```python
from build123d import *

# Parameters (mm, degrees)
F2_R     = 12.7
F3_DEPTH = 4.7625
F4_SIZE  = 1.27


with BuildPart() as f1:
    # F0 (on Front) → F1 (revolve)
    with BuildSketch(Plane.XZ):
        Polygon((-4.7625, 0), (0, 0), (0, 50.8), (-10.16, 50.8), (-10.16, 46.0375), (-4.7625, 46.0375), align=None)
    revolve(axis=Axis((0, 0, 25.4), (0, 0, -1)))

    # F2 (on face) → F3 (cut, through all)
    with BuildSketch(Plane.XY.offset(50.8)):
        Circle(F2_R)
        Polygon((-8.798818, 5.08), (0, 10.16), (8.798818, 5.08), (8.798818, -5.08), (0, -10.16), (-8.798818, -5.08), align=None, mode=Mode.SUBTRACT)
    extrude(amount=-F3_DEPTH, mode=Mode.SUBTRACT)

    # F4
    f4_edges = [f1.edges().sort_by_distance(p)[0] for p in [
        (4.7625, 0, 0),
    ]]
    chamfer(f4_edges, length=F4_SIZE)

    # F5 (on Right) → F6 (revolve, cut)
    with BuildSketch(Plane.YZ):
        Polygon((8.89, 50.8), (10.16, 49.53), (10.16, 50.8), align=None)
    revolve(axis=Axis((0, 0, 27.040424), (0, 0, 1)), mode=Mode.SUBTRACT)


solid = f1.part
```
Verification items for the finished model (mm, model axes). A direction names the side the tool comes from. Give positions to 0.01 mm unless a question says otherwise; leave off trailing zeros. Order: outer loops, then holes, each group sorted by start corner. A loop starts at its lowest first (then second) coordinate and runs counter-clockwise, first axis right, second up. Notation, with made-up numbers: (81, 51) -> (111, 51) arc R18 ccw to (111, 72) -> close; hole circle Ø3 at (25.25, 57.5). An arc over 180 degrees is marked (long way). Use a Markdown table: item, result.
1) Tool access check on faces 1 (the flat face through (-4.338, -7.656, 48.452)), 2 (the cylindrical face through (3.78, -2.9, 23.34)). Record the directions out of +Z, -Z, +X, -X, +Y, -Y that give a thin tool (end or side, any length) a straight path to the whole face; none if there is none.
Results:
| item | result |
|---|---|
| face 1 | +Z, -Z, -X, -Y |
| face 2 | -Z |
2) Section check B-B, the plane z = 30. Record the boundary of the cut face in (x, y) (1 decimal), then the cut area to 3 significant figures.
Results:
| item | result |
|---|---|
| outline | circle Ø9.5 at (0, 0) |
| area | 71.3 mm² |
3) Section check A-A, the plane y = 0. Record the boundary of the cut face in (x, z), then the cut area to 3 significant figures.
Results:
| item | result |
|---|---|
| outline | (-8.8, 46.04) -> (-4.76, 46.04) -> (-4.76, 1.27) -> (-3.49, 0) -> (3.49, 0) -> (4.76, 1.27) -> (4.76, 46.04) -> (8.8, 46.04) -> (8.8, 50.8) -> (-8.8, 50.8) -> close |
| area | 521 mm² |
4) Material ranges on probe 1 along Z at (x, y) = (7, -3); probe 2 along X at (y, z) = (-2.75, 4); probe 3 along X at (y, z) = (2.25, 16.5), recorded low to high.
Results:
| item | result |
|---|---|
| probe 1 | 46.04 to 50.8 |
| probe 2 | -3.89 to 3.89 |
| probe 3 | -4.2 to 4.2 |
5) Depth check by flat-ended pin: pin 1 Ø8 at (x, y) = (-7, -3) entering from -Z; pin 2 Ø10 at (x, z) = (5.5, 5.5) entering from +Y; pin 3 Ø8 at (x, z) = (-2.5, 43.5) entering from +Y; pin 4 Ø2 at (x, y) = (-7, 0) entering from -Z. Enter the tip coordinate at first touch or a pass-through.
Results:
| item | result |
|---|---|
| pin 1 | z = 0.12 |
| pin 2 | y = 4.74 |
| pin 3 | y = 10.16 |
| pin 4 | z = 46.04 |
